The listing builds one solid part. Answer for the finished solid, in the listing's coordinates (mm). A direction names the side the tool comes from. Round coordinates to 2 decimals unless told otherwise and drop trailing zeros. Write each loop counter-clockwise with the first axis right and the second up, starting at its lowest first coordinate (ties: lowest second). Pieces come first, ordered by that corner, then holes.
(1) For faces 1 (the face through (-68.09, 120.25, 1.52)), 2 (the face through (-54.72, -94.51, 1.48)), 3 (the face through (-1, 22, 3)), determine the directions among +Z, -Z, +X, -X, +Y, -Y from which every point of the face is accessible in a straight line to the end or side of a thin tool.
(2) A cutting plane is placed at B-B, the plane y = -108.5. Give the vertices of the cut face in (x, z).
(3) A cutting plane is placed at C-C, the plane z = 1.2. Give the number of separate pieces and of enclosed holes in the cut face, and give its area (3 significant figures).
(4) Find the intervals of material crossed by probe 1 along Y at (x, z) = (67.5, 2.2); probe 2 along Y at (x, z) = (62.5, 2.45); probe 3 along X at (y, z) = (107, 2.3), in increasing order.
(5) A cutting plane is placed at A-A, the plane x = 4.5. Give the vertices of the cut face in (y, z).
(6) Each of these flat-tipped pins is pushed along its axis until it touches: pin 1 Ø1 at (y, z) = (-63, 0.5) entering from +X; pin 2 Ø1 at (x, z) = (-43, 1) entering from -Y. Where does it stop, or does it pass through?
(7) The mould has two halves that part along Y. Classify faces 4 (the face through (-1, 22, 0)), 5 (the face through (67.981, 120.166, 1.521)), 6 (the face through (54.49, -94.28, 1.48)), 7 (the face through (69.94, 117.89, 1.52)): +Y half, -Y half, draft (parallel to the pull), parting line (faces both ways), or undercut.
Autodesk Inventor part; units mm, degrees
ref_plane "YZ Plane" through (0, 0, 0) normal (1, 0, 0) x (0, 1, 0)
ref_plane "XZ Plane" through (0, 0, 0) normal (0, 1, 0) x (-1, 0, 0)
ref_plane "XY Plane" through (0, 0, 0) normal (0, 0, 1) x (1, 0, 0)
sketch "Sketch1" plane through (0, 0, 0) normal (0, 0, 1) x (1, 0, 0)
  line L0 (-84, -130) -> (-84, 170)
  line L1 (84, -130) -> (84, 170)
  line L2 (-84, -130) -> (84, -130)
  line L3 (84, -130) -> (84, 170)
  line L4 (84, 170) -> (-84, 170)
  line L5 (-84, 170) -> (-84, -130)
  point P0 (0, 0)
extrude "Extrusion1" add sketch "Sketch1" along normal blind 3
sketch "Sketch2" plane through (0, 0, 3) normal (0, 0, 1) x (1, 0, 0)
  line L0 (-26.2712, 87.5787) -> (-28.1182, 85.2147)
  line L1 (-28.1182, 85.2147) -> (-35.9983, 91.3713)
  line L2 (-35.9983, 91.3713) -> (-34.1513, 93.7353)
  line L3 (-34.1513, 93.7353) -> (-26.2712, 87.5787)
  line L4 (-54.9105, 106.1472) -> (-53.0636, 108.5112)
  line L5 (-53.0636, 108.5112) -> (-45.1834, 102.3546)
  line L6 (-45.1834, 102.3546) -> (-47.0304, 99.9906)
  line L7 (-47.0304, 99.9906) -> (-54.9105, 106.1472)
  line L8 (-64.0957, 117.1305) -> (-65.9427, 114.7664)
  line L9 (-65.9427, 114.7664) -> (-73.8228, 120.9231)
  line L10 (-73.8228, 120.9231) -> (-71.9758, 123.2871)
  line L11 (-71.9758, 123.2871) -> (-64.0957, 117.1305)
  point P0 (0, 0)
extrude "Extrusion2" cut sketch "Sketch2" against normal blind 10
mirror "Mirror1" about plane through (0, 0, 0) normal (1, 0, 0) of "Extrusion2"
sketch "Sketch3" plane through (0, 0, 3) normal (0, 0, 1) x (1, 0, 0)
  line L0 (44, 18) -> (41, 18)
  line L1 (41, 18) -> (41, 33)
  line L2 (41, 33) -> (44, 33)
  line L3 (44, 33) -> (44, 18)
  line L4 (44, 53) -> (41, 53)
  line L5 (41, 53) -> (41, 68)
  line L6 (41, 68) -> (44, 68)
  line L7 (44, 68) -> (44, 53)
  line L8 (-41, 18) -> (-44, 18)
  line L9 (-44, 18) -> (-44, 33)
  line L10 (-44, 33) -> (-41, 33)
  line L11 (-41, 33) -> (-41, 18)
  line L12 (-41, 53) -> (-44, 53)
  line L13 (-44, 53) -> (-44, 68)
  line L14 (-44, 68) -> (-41, 68)
  line L15 (-41, 68) -> (-41, 53)
  point P0 (0, 0)
extrude "Extrusion3" cut sketch "Sketch3" against normal blind 10
sketch "Sketch4" plane through (0, 0, 3) normal (0, 0, 1) x (1, 0, 0)
  line L0 (84, -130) -> (84, 170)
  line L1 (84, 170) -> (87, 170)
  line L2 (87, 170) -> (87, -130)
  line L3 (87, -130) -> (84, -130)
  line L4 (84, -130) -> (84, 170)
  line L5 (-84, -130) -> (84, -130)
  line L6 (0, 0) -> (0, -130) construction
  line L7 (-84, -130) -> (-84, 170)
  line L8 (-84, 170) -> (-87, 170)
  line L9 (-87, 170) -> (-87, -130)
  line L10 (-87, -130) -> (-84, -130)
  line L11 (-84, -130) -> (-84, 170)
  dimension "d6" = 3
extrude "Extrusion4" add sketch "Sketch4" against normal up to surface (3 mm away)
sketch "Sketch5" plane through (0, 0, 3) normal (0, 0, 1) x (1, 0, 0)
  line L0 (-87, 170) -> (-84, 170)
  line L1 (-84, 170) -> (-84, 70)
  line L2 (-84, 70) -> (-87, 70)
  line L3 (-87, 70) -> (-87, 170)
  line L4 (-84, -130) -> (-87, -130)
  line L5 (-87, -130) -> (-87, -30)
  line L6 (-87, -30) -> (-84, -30)
  line L7 (-84, -30) -> (-84, -130)
  line L8 (84, 170) -> (87, 170)
  line L9 (87, 170) -> (87, 70)
  line L10 (87, 70) -> (84, 70)
  line L11 (84, 70) -> (84, 170)
  line L12 (87, -130) -> (84, -130)
  line L13 (84, -130) -> (84, -30)
  line L14 (84, -30) -> (87, -30)
  line L15 (87, -30) -> (87, -130)
  point P0 (0, 0)
extrude "Extrusion5" cut sketch "Sketch5" against normal blind 10
sketch "Sketch6" plane through (0, 0, 3) normal (0, 0, 1) x (1, 0, 0)
  line L0 (84, -130) -> (-84, -130)
  line L1 (-59, -130) -> (59, -130)
  line L2 (59, -130) -> (59, -90)
  line L3 (59, -90) -> (-59, -90)
  line L4 (-59, -90) -> (-59, -130)
  line L5 (84, -130) -> (84, -30)
  line L6 (-84, -30) -> (-84, -130)
  point P0 (0, 0)
  dimension "d11" = 40
  dimension "d12" = 25
  dimension "d13" = 25
extrude "Extrusion6" cut sketch "Sketch6" against normal blind 10
fillet "Fillet1" radius 15 2 edges at (-59, -90, 1.5) (59, -90, 1.5)
sketch "Sketch8" plane through (0, 0, 3) normal (0, 0, 1) x (1, 0, 0)
  line L0 (73, -23.2) -> (73, -20)
  line L1 (73, -20) -> (79, -20)
  line L2 (79, -20) -> (79, -23.2)
  line L3 (79, -23.2) -> (73, -23.2)
  line L4 (22.5, -23.2) -> (22.5, -20)
  line L5 (22.5, -20) -> (28.5, -20)
  line L6 (28.5, -20) -> (28.5, -23.2)
  line L7 (28.5, -23.2) -> (22.5, -23.2)
  line L8 (32.5, -23.2) -> (35.5, -23.2)
  line L9 (35.5, -23.2) -> (35.5, -20)
  line L10 (32.5, -20) -> (35.5, -20)
  line L11 (32.5, -23.2) -> (32.5, -20)
  line L12 (66, -23.2) -> (69, -23.2)
  line L13 (69, -23.2) -> (69, -20)
  line L14 (66, -20) -> (69, -20)
  line L15 (66, -23.2) -> (66, -20)
  line L16 (32.5, -20) -> (35.5, -23.2) construction
  line L17 (69, -23.2) -> (66, -20) construction
  circle A0 centre (67.5, -21.6) radius 1.5
  circle A1 centre (34, -21.6) radius 1.5
  point P0 (0, 0)
  dimension "d33" = 3
  dimension "d34" = 3
extrude "Extrusion8" cut sketch "Sketch8" against normal blind 10 contours L0 L1 L2 L3 | L4 L5 L6 L7 | A1 | A0
sketch "Sketch7" plane through (0, 0, 3) normal (0, 0, 1) x (1, 0, 0)
  line L0 (44, 33) -> (44, 18)
  line L1 (44, 18) -> (41, 18)
  line L2 (54.25, 10) -> (73.75, 10)
  line L3 (73.75, 10) -> (73.75, 22.55)
  line L4 (73.75, 22.55) -> (54.25, 22.55)
  line L5 (54.25, 22.55) -> (54.25, 10)
  line L6 (54.25, 10) -> (73.75, 22.55) construction
  line L7 (73.75, 10) -> (54.25, 22.55) construction
  line L8 (64, 19.1981) -> (64, 44.4042) construction
  line L9 (87, -30) -> (87, 70) construction
  line L10 (84, -130) -> (84, -30)
  line L11 (44, 18) -> (44, 33) construction
  line L12 (44, 19.1981) -> (84, 19.1981) construction
  circle A0 centre (50.75, -21.6) radius 5
  line L13 (28.5, -20) -> (28.5, -23.2) construction
  line L14 (73, -23.2) -> (73, -20) construction
  line L15 (28.5, -23.2) -> (28.5, -20) construction
  line L16 (28.5, -21.6) -> (73, -21.6) construction
  point P0 (0, 0)
  point P1 (64, 16.275)
  point P2 (64, 16.275)
  dimension "d23" = 12.55
  dimension "d24" = 19.5
  dimension "d29" = 8
  dimension "d30" = 10
extrude "Extrusion7" cut sketch "Sketch7" against normal blind 10
sketch "Sketch9" plane through (0, 0, 3) normal (0, 0, 1) x (1, 0, 0)
  line L0 (25, 3) -> (25, 0)
  line L1 (25, 0) -> (-25, 0)
  line L2 (-25, 0) -> (-25, 3)
  line L3 (-25, 3) -> (25, 3)
  point P0 (0, 0)
extrude "Extrusion9" cut sketch "Sketch9" against normal blind 10
properties part number "Pared_Frontal"
Solutions:
1. face 1: +Z, -Z
1. face 2: +Z, -Z, -Y
1. face 3: +Z, +X, -X, +Y, -Y
2. outline: (-84, 0) - (-59, 0) - (-59, 3) - (-84, 3) - close; (59, 0) - (84, 0) - (84, 3) - (59, 3) - close
3. separate pieces: 1
3. enclosed holes: 17
3. area: 45,500 mm2
4. probe 1: y = -130 to -23.1, -20.1 to 10, 22.55 to 115.98, 119.79 to 170
4. probe 2: y = -130 to 10, 22.55 to 170
4. probe 3: x = -84 to -54.24, -51.13 to 51.13, 54.24 to 84
5. outline: (-90, 0) - (0, 0) - (0, 3) - (-90, 3) - close; (3, 0) - (170, 0) - (170, 3) - (3, 3) - close
6. pin 1: stops at x = 84
6. pin 2: stops at y = -90
7. face 4: draft
7. face 5: undercut
7. face 6: -Y half
7. face 7: undercut
